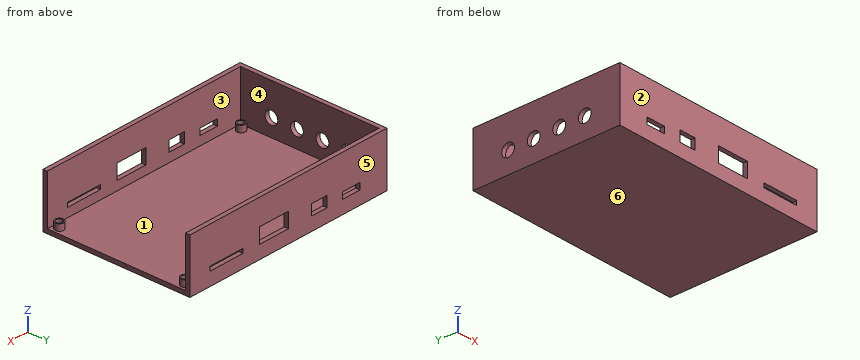
Autodesk Fusion 360 part; units mm, degrees
sketch "Sketch1" plane through (0, 0, 0) normal (0, 0, 1) x (1, 0, 0)
  line L0 (0, 0) -> (100, 0)
  line L1 (100, 0) -> (100, -65)
  line L2 (100, -65) -> (0, -65)
  line L3 (0, -65) -> (0, 0)
  dimension "d1" = 100
  dimension "d2" = 65
extrude "Extrude1" add sketch "Sketch1" along normal blind 2
sketch "Sketch2" plane through (0, 0, 2) normal (0, 0, 1) x (-1, 0, 0)
  line L0 (0, 65) -> (-100, 65)
  line L1 (-100, 65) -> (-100, 0)
  line L2 (-100, 0) -> (0, 0)
  line L3 (0, 0) -> (0, 65)
  line L4 (0, 65) -> (-120, 65)
  line L5 (-120, 65) -> (-210, 65)
  line L6 (-210, 65) -> (-290, 65)
  line L7 (-290, 65) -> (-370, 65)
  line L8 (-370, 65) -> (-490, 65)
  line L9 (-490, 65) -> (-640, 65)
  line L10 (-640, 65) -> (-725, 65)
  line L11 (-725, 65) -> (-895, 65)
  line L12 (-895, 65) -> (-1000, 65)
  line L13 (0, 0) -> (-1.5, 0)
  line L14 (-1.5, 0) -> (-1.5, 1.5)
  line L15 (-1.5, 1.5) -> (-1.5, 3)
  line L16 (-1.5, 3) -> (-3, 3)
  circle A0 centre (-3, 3) radius 1.5
  circle A1 centre (-3, 3) radius 2
  dimension "d5" = 120
  dimension "d6" = 90
  dimension "d7" = 80
  dimension "d8" = 80
  dimension "d9" = 120
  dimension "d10" = 150
  dimension "d11" = 85
  dimension "d12" = 170
  dimension "d13" = 105
  dimension "d14" = 1.5
  dimension "d15" = 1.5
  dimension "d16" = 1.5
  dimension "d17" = 1.5
  dimension "d18" = 3
extrude "Extrude2" add sketch "Sketch2" along normal blind 3 contours A1
pattern_linear "R-Pattern2" count 2 spacing 94 along (1, 0, 0) count 2 spacing 59 along (0, -1, 0) of "Extrude2"
sketch "Sketch4" plane through (0, 0, 0) normal (0, 0, -1) x (1, 0, 0)
  line L0 (100, 65) -> (0, 65)
  line L1 (0, 65) -> (0, 0)
  line L2 (0, 0) -> (100, 0)
  line L3 (100, 0) -> (100, 65)
  line L4 (0, 0) -> (-2, 0)
  line L5 (-2, 0) -> (-2, 65)
  line L6 (-2, 65) -> (0, 65)
  line L7 (0, 65) -> (0, 0)
  line L8 (-2, 65) -> (100, 65)
  line L9 (100, 65) -> (100, 67)
  line L10 (100, 67) -> (-2, 67)
  line L11 (-2, 67) -> (-2, 65)
  dimension "d37" = 2
  dimension "d38" = 2
extrude "Extrude6" add sketch "Sketch4" against normal blind 25 contours L0 L6 L8 L9 L10 L11 | L1 L4 L5 L6 L7 L8
sketch "Sketch5" plane through (0, -67, 0) normal (0, -1, 0) x (1, 0, 0)
  line L0 (-2, 0) -> (100, 0)
  line L1 (100, 0) -> (100, 25)
  line L2 (100, 25) -> (-2, 25)
  line L3 (-2, 25) -> (-2, 0)
  line L4 (0, 25) -> (0, 0) construction
  line L5 (0, 5) -> (100, 5) construction
  line L6 (0, 5) -> (100, 5)
  line L7 (100, 5) -> (100, 6.15)
  line L8 (100, 6.15) -> (0, 6.15)
  line L9 (0, 6.15) -> (0, 5)
  line L10 (0, 6.15) -> (12, 6.15)
  line L11 (12, 6.15) -> (21, 6.15)
  line L12 (21, 6.15) -> (21, 9.15)
  line L13 (21, 9.15) -> (12, 9.15)
  line L14 (12, 9.15) -> (12, 6.15)
  line L15 (21, 6.15) -> (29, 6.15)
  line L16 (29, 6.15) -> (37, 6.15)
  line L17 (37, 6.15) -> (37, 11.15)
  line L18 (37, 11.15) -> (29, 11.15)
  line L19 (29, 11.15) -> (29, 6.15)
  line L20 (37, 6.15) -> (49, 6.15)
  line L21 (49, 6.15) -> (64, 6.15)
  line L22 (64, 6.15) -> (64, 13.15)
  line L23 (64, 13.15) -> (49, 13.15)
  line L24 (49, 13.15) -> (49, 6.15)
  line L25 (64, 6.15) -> (72.5, 6.15)
  line L26 (72.5, 6.15) -> (89.5, 6.15)
  line L27 (89.5, 6.15) -> (89.5, 8.15)
  line L28 (89.5, 8.15) -> (72.5, 8.15)
  line L29 (72.5, 8.15) -> (72.5, 6.15)
  line L30 (89.5, 6.15) -> (100, 6.15)
  dimension "d41" = 1.15
  dimension "d42" = 12
  dimension "d43" = 9
  dimension "d44" = 3
  dimension "d45" = 8
  dimension "d46" = 8
  dimension "d47" = 5
  dimension "d48" = 12
  dimension "d49" = 15
  dimension "d50" = 7
  dimension "d51" = 8.5
  dimension "d52" = 17
  dimension "d53" = 2
extrude "Extrude7" cut sketch "Sketch5" against normal up to surface (2 mm away) contours L8 L26 L27 L28 L29 | L8 L11 L12 L13 L14 | L8 L21 L22 L23 L24 | L8 L16 L17 L18 L19
sketch "Sketch6" plane through (-2, 0, 0) normal (-1, 0, 0) x (0, -1, 0)
  line L0 (0, 0) -> (67, 0)
  line L1 (67, 0) -> (67, 25)
  line L2 (67, 25) -> (0, 25)
  line L3 (0, 25) -> (0, 0)
  line L4 (65, 25) -> (65, 0)
  line L5 (67, 5) -> (0, 5)
  line L6 (67, 5) -> (0, 5)
  line L7 (0, 5) -> (0, 6.15)
  line L8 (0, 6.15) -> (67, 6.15) construction
  line L9 (67, 6.15) -> (67, 5)
  line L10 (65, 5) -> (65, 10)
  line L11 (65, 10) -> (0, 10)
  line L12 (65, 10) -> (50.5, 10)
  circle A0 centre (50.5, 10) radius 3
  line L13 (50.5, 10) -> (38.5, 10)
  circle A1 centre (38.5, 10) radius 3
  line L14 (38.5, 10) -> (26.5, 10)
  circle A2 centre (26.5, 10) radius 3
  line L15 (26.5, 10) -> (14.5, 10)
  circle A3 centre (14.5, 10) radius 3
  dimension "d56" = 67
  dimension "d57" = 1.15
  dimension "d58" = 5
  dimension "d59" = 14.5
  dimension "d60" = 6
  dimension "d61" = 12
  dimension "d62" = 12
  dimension "d63" = 12
ref_plane "WorkPlane1" through (50, -32.5, 13.5) normal (0, 1, 0) x (-1, 0, 0)
mirror "Mirror1" about plane through (50, -32.5, 13.5) normal (0, 1, 0) of "Extrude6"
extrude "Extrude8" cut sketch "Sketch6" against normal up to surface (2 mm away) contours L11 L12 A0 L13 | L11 L12 A0 L13 | L11 L15 A3 | L11 L15 A3 | L11 L13 A1 L14 | L11 L13 A1 L14 | L11 L14 A2 L15 | L11 L14 A2 L15
mirror "Mirror2" about plane through (50, -32.5, 13.5) normal (0, 1, 0) of "Extrude7"
Here's how the part is built. I have some questions about the finished solid (model axes, mm). Face numbers are marked on the shaded views. A direction names the side the tool comes from. Coordinates: 2 decimals unless noted, no trailing zeros. Write each loop counter-clockwise with the first axis right and the second up, starting at its lowest first coordinate (ties: lowest second). Pieces come first, ordered by that corner, then holes. Notation, with made-up numbers: (-14.75, -22) -> (35.25, -22) arc R32 ccw to (35.25, 17) -> close; hole circle Ø11 at (-5, 58.5). An arc over 180 degrees is marked (long way). Use a Markdown table: item, result. Add a question column.
(1) If we section it at A-A, the plane y = -50.5: Write out the boundary of the cut face in (x, z).
(2) Please list where these lines run through material, in increasing order: line 1 (Y direction, x = -0.75, z = 10); line 2 (X direction, y = -3, z = 4.45); line 3 (Y direction, x = 91.5, z = 7.25).
(3) For the marked faces 1, 2 and 3, which set-ups out of +Z, -Z, +X, -X, +Y, -Y let a thin tool reach every point of the face, with its end or its side?
(4) If we section it at D-D, the plane z = 21: Write out the boundary of the cut face in (x, y).
(5) I'm going to push flat-ended pins straight in: P1, Ø1, axis at y = -18.5, z = 19, coming from the +X side; P2, Ø1.2, axis at x = 96, y = -61, coming from the +Z side; P3, Ø10, axis at x = 74.5, y = -18, coming from the +Z side. Where does each tip first touch, or does it pass through?
(6) If we section it at C-C, the plane x = 3: Write out the boundary of the cut face in (y, z).
(7) We'd pull the mould along Y, two halves only. Please class the marked faces 4, 5 and 6: +Y half, -Y half, draft (parallel to the pull), parting line (faces both ways), or undercut.
(8) If we section it at B-B, the plane x = 80: Write out the boundary of the cut face in (y, z), and give its area (3 significant figures).
Outcome:
| question | item | result |
|---|---|---|
| 1 | outline | (-2, 0) -> (100, 0) -> (100, 2) -> (0, 2) -> (0, 7) -> (-2, 7) -> close; (-2, 13) -> (0, 13) -> (0, 25) -> (-2, 25) -> close |
| 2 | line 1 | y = -67 to -53.5, -47.5 to -41.5, -35.5 to -29.5, -23.5 to -17.5, -11.5 to 2 |
| 2 | line 2 | x = -2 to 0, 1 to 1.5, 4.5 to 5, 95 to 95.5, 98.5 to 99 |
| 2 | line 3 | y = -67 to -65, 0 to 2 |
| 3 | face 1 | +Z |
| 3 | face 2 | +Z, -Z, +X, -X, -Y |
| 3 | face 3 | +Z, +X |
| 4 | outline | (-2, -67) -> (100, -67) -> (100, -65) -> (0, -65) -> (0, 0) -> (100, 0) -> (100, 2) -> (-2, 2) -> close |
| 5 | P1 | stops at x = 0 |
| 5 | P2 | stops at z = 5 |
| 5 | P3 | stops at z = 2 |
| 6 | outline | (-67, 0) -> (2, 0) -> (2, 25) -> (0, 25) -> (0, 2) -> (-1, 2) -> (-1, 5) -> (-1.5, 5) -> (-1.5, 2) -> (-4.5, 2) -> (-4.5, 5) -> (-5, 5) -> (-5, 2) -> (-60, 2) -> (-60, 5) -> (-60.5, 5) -> (-60.5, 2) -> (-63.5, 2) -> (-63.5, 5) -> (-64, 5) -> (-64, 2) -> (-65, 2) -> (-65, 25) -> (-67, 25) -> close |
| 7 | face 4 | undercut |
| 7 | face 5 | +Y half |
| 7 | face 6 | draft |
| 8 | outline | (-67, 0) -> (2, 0) -> (2, 6.15) -> (0, 6.15) -> (0, 2) -> (-65, 2) -> (-65, 6.15) -> (-67, 6.15) -> close; (-67, 8.15) -> (-65, 8.15) -> (-65, 25) -> (-67, 25) -> close; (0, 8.15) -> (2, 8.15) -> (2, 25) -> (0, 25) -> close |
| 8 | area | 222 mm^2 |
